Part model, mm, in its own coordinate system. A direction names the side the tool comes from. Round coordinates to 2 decimals unless told otherwise and drop trailing zeros. Loops run counter-clockwise (first coordinate to the right, second up) from the corner with the lowest first, then second, coordinate; pieces in that order, holes last. Notation, with made-up numbers: M -25.5,16.5 L -0.5,16.5 A27 cw -0.5,51.5 Z; hole C 24,45 d11. An arc over 180 degrees is marked long. Put each result on its own line as item: value. Start each with the question number.
1) Slice it at B-B on y = 13.97. State how many separate pieces and enclosed holes the cut face has, then the cut area to 3 significant figures.
2) Probe line 1 along X through (y, z) = (3.5, 145); line 2 along Y through (x, z) = (45, 132.5); line 3 along X through (y, z) = (1.45, 419.1). List the from-to ranges inside material, lowest first.
3) Pull direction Z, two halves, no side cores. Call faces 1 (the flat face through (41.69, 1.25, 8.85)), 2 (the flat face through (25, 2.54, 213)), 3 (the flat face through (26.553, 1.252, 88.849)): +Z half, -Z half, draft (parallel to the pull), parting line (faces both ways), or undercut.
4) Slice it at C-C on z = 76. Give the cut face in (x, y), then the cut area to 3 significant figures.
5) Which spindle directions (+Z, -Z, +X, -X, +Y, -Y) get a long thin tool onto all of the face, cutting with end or side? Do faces 4 (the flat face through (26, 0, 213)), 5 (the flat face through (2.54, 14, 213)), 6 (the flat face through (26.553, 1.252, 355.549)). Say none if no direction does.
6) Slice it at A-A on z = 303. Give the cut face in (x, y), then the cut area to 3 significant figures.
7) Slice it at D-D on z = 169.5. Give the cut face in (x, y), then the cut area to 3 significant figures.
8) Drop flat-ended pins along their axis: pin 1 Ø12 at (x, y) = (45, 9) entering from -Z; pin 2 Ø10 at (x, z) = (44.5, 307) entering from -Y; pin 3 Ø1.3 at (x, y) = (17, 1.5) entering from -Z; pin 4 Ø8 at (x, y) = (9.5, 6) entering from +Z. Give the stop position or say it passes through.
```python
from build123d import *

# Parameters (mm, degrees)
BOSS_EXTRUDE1_DEPTH   = 431.8
SKETCH2_W             = 50.8
SKETCH2_H             = 38.1
TABS_DEPTH            = 22.86
HOLES_REACH           = 4.54
SKETCH3_R             = 2.5796875
SLOTS_DEPTH           = 51.8
TRIG_HOLES_REACH      = 27.4
TAB_CORNER_CUTS_REACH = 27.4


with BuildPart() as part:
    # Sketch1 → Boss-Extrude1 (new body)
    with BuildSketch(Plane.XY):
        Polygon((48.26, 2.54), (48.26, 25.4), (50.8, 25.4), (50.8, 0), (0, 0), (0, 25.4), (2.54, 25.4), (2.54, 2.54), align=None)
    extrude(amount=BOSS_EXTRUDE1_DEPTH)

    # Sketch2 → Tabs (cut)
    with BuildSketch(Plane(origin=(0, 25.4, 0), x_dir=(1, 0, 0), z_dir=(0, 1, 0))):
        with Locations((25.4, -412.75)):
            Rectangle(SKETCH2_W, SKETCH2_H)
        with Locations((25.4, -19.05)):
            Rectangle(SKETCH2_W, SKETCH2_H)
    extrude(amount=-TABS_DEPTH, mode=Mode.SUBTRACT)

    # Sketch3 → Holes (cut, up to next)
    with BuildSketch(Plane(origin=(0, 2.54, 0), x_dir=(1, 0, 0), z_dir=(0, 1, 0)), mode=Mode.PRIVATE) as holes_sk1:
        with Locations((25.4, -419.1)):
            Circle(SKETCH3_R)
    holes_tool1 = extrude(holes_sk1.sketch, amount=-HOLES_REACH, mode=Mode.PRIVATE) & part.part
    add(holes_tool1.solids().sort_by_distance((25.4, 2.54, 419.1))[0], mode=Mode.SUBTRACT)
    # Sketch3 → Holes (cut, up to next)
    with BuildSketch(Plane(origin=(0, 2.54, 0), x_dir=(1, 0, 0), z_dir=(0, 1, 0)), mode=Mode.PRIVATE) as holes_sk2:
        with Locations((25.4, -12.7)):
            Circle(SKETCH3_R)
    holes_tool2 = extrude(holes_sk2.sketch, amount=-HOLES_REACH, mode=Mode.PRIVATE) & part.part
    add(holes_tool2.solids().sort_by_distance((25.4, 2.54, 12.7))[0], mode=Mode.SUBTRACT)

    # Sketch4 → Slots (cut, through all)
    with BuildSketch(Plane(origin=(50.8, 0, 0), x_dir=(0, 0, -1), z_dir=(1, 0, 0))):
        with BuildLine():
            Line((-57.15, 7.62), (-117.475, 7.62))
            ThreePointArc((-117.475, 7.62), (-123.825, 13.97), (-117.475, 20.32))
            Line((-117.475, 20.32), (-57.15, 20.32))
            ThreePointArc((-57.15, 20.32), (-50.8, 13.97), (-57.15, 7.62))
        make_face()
        with BuildLine():
            Line((-142.875, 7.62), (-203.2, 7.62))
            ThreePointArc((-203.2, 7.62), (-209.55, 13.97), (-203.2, 20.32))
            Line((-203.2, 20.32), (-142.875, 20.32))
            ThreePointArc((-142.875, 20.32), (-136.525, 13.97), (-142.875, 7.62))
        make_face()
        with BuildLine():
            Line((-228.6, 7.62), (-288.925, 7.62))
            ThreePointArc((-288.925, 7.62), (-295.275, 13.97), (-288.925, 20.32))
            Line((-288.925, 20.32), (-228.6, 20.32))
            ThreePointArc((-228.6, 20.32), (-222.25, 13.97), (-228.6, 7.62))
        make_face()
        with BuildLine():
            Line((-314.325, 7.62), (-374.65, 7.62))
            ThreePointArc((-374.65, 7.62), (-381, 13.97), (-374.65, 20.32))
            Line((-374.65, 20.32), (-314.325, 20.32))
            ThreePointArc((-314.325, 20.32), (-307.975, 13.97), (-314.325, 7.62))
        make_face()
    extrude(amount=-SLOTS_DEPTH, mode=Mode.SUBTRACT)

    # Sketch5 → Trig_Holes (cut, up to next)
    with BuildSketch(Plane.XZ, mode=Mode.PRIVATE) as trig_holes_sk1:
        with BuildLine():
            Line((41.275, 52.3875), (12.7, 52.3875))
            ThreePointArc((12.7, 52.3875), (9.860193669, 54.142596834), (10.16, 57.4675))
            Line((10.16, 57.4675), (38.735, 95.5675))
            ThreePointArc((38.735, 95.5675), (42.279023157, 96.674569471), (44.45, 93.6625))
            Line((44.45, 93.6625), (44.45, 55.5625))
            ThreePointArc((44.45, 55.5625), (43.52006403, 53.31743597), (41.275, 52.3875))
        make_face()
    trig_holes_tool1 = extrude(trig_holes_sk1.sketch, amount=-TRIG_HOLES_REACH, mode=Mode.PRIVATE) & part.part
    add(trig_holes_tool1.solids().sort_by_distance((31.731608, 0, 68.958649))[0], mode=Mode.SUBTRACT)
    # Sketch5 → Trig_Holes (cut, up to next)
    with BuildSketch(Plane.XZ, mode=Mode.PRIVATE) as trig_holes_sk2:
        with BuildLine():
            Line((9.525, 112.7125), (38.1, 112.7125))
            ThreePointArc((38.1, 112.7125), (40.939806331, 110.957403166), (40.64, 107.6325))
            Line((40.64, 107.6325), (12.065, 69.5325))
            ThreePointArc((12.065, 69.5325), (8.520976843, 68.425430529), (6.35, 71.4375))
            Line((6.35, 71.4375), (6.35, 109.5375))
            ThreePointArc((6.35, 109.5375), (7.27993597, 111.78256403), (9.525, 112.7125))
        make_face()
    trig_holes_tool2 = extrude(trig_holes_sk2.sketch, amount=-TRIG_HOLES_REACH, mode=Mode.PRIVATE) & part.part
    add(trig_holes_tool2.solids().sort_by_distance((19.068392, 0, 96.141351))[0], mode=Mode.SUBTRACT)
    # Sketch5 → Trig_Holes (cut, up to next)
    with BuildSketch(Plane.XZ, mode=Mode.PRIVATE) as trig_holes_sk3:
        with BuildLine():
            Line((41.275, 119.0625), (12.7, 119.0625))
            ThreePointArc((12.7, 119.0625), (9.860193669, 120.817596834), (10.16, 124.1425))
            Line((10.16, 124.1425), (38.735, 162.2425))
            ThreePointArc((38.735, 162.2425), (42.279023157, 163.349569471), (44.45, 160.3375))
            Line((44.45, 160.3375), (44.45, 122.2375))
            ThreePointArc((44.45, 122.2375), (43.52006403, 119.99243597), (41.275, 119.0625))
        make_face()
    trig_holes_tool3 = extrude(trig_holes_sk3.sketch, amount=-TRIG_HOLES_REACH, mode=Mode.PRIVATE) & part.part
    add(trig_holes_tool3.solids().sort_by_distance((31.731608, 0, 135.633649))[0], mode=Mode.SUBTRACT)
    # Sketch5 → Trig_Holes (cut, up to next)
    with BuildSketch(Plane.XZ, mode=Mode.PRIVATE) as trig_holes_sk4:
        with BuildLine():
            Line((9.525, 179.3875), (38.1, 179.3875))
            ThreePointArc((38.1, 179.3875), (40.939806331, 177.632403166), (40.64, 174.3075))
            Line((40.64, 174.3075), (12.065, 136.2075))
            ThreePointArc((12.065, 136.2075), (8.520976843, 135.100430529), (6.35, 138.1125))
            Line((6.35, 138.1125), (6.35, 176.2125))
            ThreePointArc((6.35, 176.2125), (7.27993597, 178.45756403), (9.525, 179.3875))
        make_face()
    trig_holes_tool4 = extrude(trig_holes_sk4.sketch, amount=-TRIG_HOLES_REACH, mode=Mode.PRIVATE) & part.part
    add(trig_holes_tool4.solids().sort_by_distance((19.068392, 0, 162.816351))[0], mode=Mode.SUBTRACT)
    # Sketch5 → Trig_Holes (cut, up to next)
    with BuildSketch(Plane.XZ, mode=Mode.PRIVATE) as trig_holes_sk5:
        with BuildLine():
            Line((41.275, 185.7375), (12.7, 185.7375))
            ThreePointArc((12.7, 185.7375), (9.860193669, 187.492596834), (10.16, 190.8175))
            Line((10.16, 190.8175), (38.735, 228.9175))
            ThreePointArc((38.735, 228.9175), (42.279023157, 230.024569471), (44.45, 227.0125))
            Line((44.45, 227.0125), (44.45, 188.9125))
            ThreePointArc((44.45, 188.9125), (43.52006403, 186.66743597), (41.275, 185.7375))
        make_face()
    trig_holes_tool5 = extrude(trig_holes_sk5.sketch, amount=-TRIG_HOLES_REACH, mode=Mode.PRIVATE) & part.part
    add(trig_holes_tool5.solids().sort_by_distance((31.731608, 0, 202.308649))[0], mode=Mode.SUBTRACT)
    # Sketch5 → Trig_Holes (cut, up to next)
    with BuildSketch(Plane.XZ, mode=Mode.PRIVATE) as trig_holes_sk6:
        with BuildLine():
            Line((9.525, 246.0625), (38.1, 246.0625))
            ThreePointArc((38.1, 246.0625), (40.939806331, 244.307403166), (40.64, 240.9825))
            Line((40.64, 240.9825), (12.065, 202.8825))
            ThreePointArc((12.065, 202.8825), (8.520976843, 201.775430529), (6.35, 204.7875))
            Line((6.35, 204.7875), (6.35, 242.8875))
            ThreePointArc((6.35, 242.8875), (7.27993597, 245.13256403), (9.525, 246.0625))
        make_face()
    trig_holes_tool6 = extrude(trig_holes_sk6.sketch, amount=-TRIG_HOLES_REACH, mode=Mode.PRIVATE) & part.part
    add(trig_holes_tool6.solids().sort_by_distance((19.068392, 0, 229.491351))[0], mode=Mode.SUBTRACT)
    # Sketch5 → Trig_Holes (cut, up to next)
    with BuildSketch(Plane.XZ, mode=Mode.PRIVATE) as trig_holes_sk7:
        with BuildLine():
            Line((41.275, 252.4125), (12.7, 252.4125))
            ThreePointArc((12.7, 252.4125), (9.860193669, 254.167596834), (10.16, 257.4925))
            Line((10.16, 257.4925), (38.735, 295.5925))
            ThreePointArc((38.735, 295.5925), (42.279023157, 296.699569471), (44.45, 293.6875))
            Line((44.45, 293.6875), (44.45, 255.5875))
            ThreePointArc((44.45, 255.5875), (43.52006403, 253.34243597), (41.275, 252.4125))
        make_face()
    trig_holes_tool7 = extrude(trig_holes_sk7.sketch, amount=-TRIG_HOLES_REACH, mode=Mode.PRIVATE) & part.part
    add(trig_holes_tool7.solids().sort_by_distance((31.731608, 0, 268.983649))[0], mode=Mode.SUBTRACT)
    # Sketch5 → Trig_Holes (cut, up to next)
    with BuildSketch(Plane.XZ, mode=Mode.PRIVATE) as trig_holes_sk8:
        with BuildLine():
            Line((9.525, 312.7375), (38.1, 312.7375))
            ThreePointArc((38.1, 312.7375), (40.939806331, 310.982403166), (40.64, 307.6575))
            Line((40.64, 307.6575), (12.065, 269.5575))
            ThreePointArc((12.065, 269.5575), (8.520976843, 268.450430529), (6.35, 271.4625))
            Line((6.35, 271.4625), (6.35, 309.5625))
            ThreePointArc((6.35, 309.5625), (7.27993597, 311.80756403), (9.525, 312.7375))
        make_face()
    trig_holes_tool8 = extrude(trig_holes_sk8.sketch, amount=-TRIG_HOLES_REACH, mode=Mode.PRIVATE) & part.part
    add(trig_holes_tool8.solids().sort_by_distance((19.068392, 0, 296.166351))[0], mode=Mode.SUBTRACT)
    # Sketch5 → Trig_Holes (cut, up to next)
    with BuildSketch(Plane.XZ, mode=Mode.PRIVATE) as trig_holes_sk9:
        with BuildLine():
            Line((41.275, 319.0875), (12.7, 319.0875))
            ThreePointArc((12.7, 319.0875), (9.860193669, 320.842596834), (10.16, 324.1675))
            Line((10.16, 324.1675), (38.735, 362.2675))
            ThreePointArc((38.735, 362.2675), (42.279023157, 363.374569471), (44.45, 360.3625))
            Line((44.45, 360.3625), (44.45, 322.2625))
            ThreePointArc((44.45, 322.2625), (43.52006403, 320.01743597), (41.275, 319.0875))
        make_face()
    trig_holes_tool9 = extrude(trig_holes_sk9.sketch, amount=-TRIG_HOLES_REACH, mode=Mode.PRIVATE) & part.part
    add(trig_holes_tool9.solids().sort_by_distance((31.731608, 0, 335.658649))[0], mode=Mode.SUBTRACT)
    # Sketch5 → Trig_Holes (cut, up to next)
    with BuildSketch(Plane.XZ, mode=Mode.PRIVATE) as trig_holes_sk10:
        with BuildLine():
            Line((9.525, 379.4125), (38.1, 379.4125))
            ThreePointArc((38.1, 379.4125), (40.939806331, 377.657403166), (40.64, 374.3325))
            Line((40.64, 374.3325), (12.065, 336.2325))
            ThreePointArc((12.065, 336.2325), (8.520976843, 335.125430529), (6.35, 338.1375))
            Line((6.35, 338.1375), (6.35, 376.2375))
            ThreePointArc((6.35, 376.2375), (7.27993597, 378.48256403), (9.525, 379.4125))
        make_face()
    trig_holes_tool10 = extrude(trig_holes_sk10.sketch, amount=-TRIG_HOLES_REACH, mode=Mode.PRIVATE) & part.part
    add(trig_holes_tool10.solids().sort_by_distance((19.068392, 0, 362.841351))[0], mode=Mode.SUBTRACT)

    # Sketch6 → Tab_Corner_Cuts (cut, up to next)
    with BuildSketch(Plane.XZ, mode=Mode.PRIVATE) as tab_corner_cuts_sk1:
        Polygon((32.839487758, 0), (50.8, 17.960512242), (50.8, 0), align=None)
    tab_corner_cuts_tool1 = extrude(tab_corner_cuts_sk1.sketch, amount=-TAB_CORNER_CUTS_REACH, mode=Mode.PRIVATE) & part.part
    add(tab_corner_cuts_tool1.solids().sort_by_distance((44.813163, 0, 5.986837))[0], mode=Mode.SUBTRACT)
    # Sketch6 → Tab_Corner_Cuts (cut, up to next)
    with BuildSketch(Plane.XZ, mode=Mode.PRIVATE) as tab_corner_cuts_sk2:
        Polygon((17.960512242, 0), (0, 17.960512242), (0, 0), align=None)
    tab_corner_cuts_tool2 = extrude(tab_corner_cuts_sk2.sketch, amount=-TAB_CORNER_CUTS_REACH, mode=Mode.PRIVATE) & part.part
    add(tab_corner_cuts_tool2.solids().sort_by_distance((5.986837, 0, 5.986837))[0], mode=Mode.SUBTRACT)
    # Sketch6 → Tab_Corner_Cuts (cut, up to next)
    with BuildSketch(Plane.XZ, mode=Mode.PRIVATE) as tab_corner_cuts_sk3:
        Polygon((32.839487758, 431.8), (50.8, 413.839487758), (50.8, 431.8), align=None)
    tab_corner_cuts_tool3 = extrude(tab_corner_cuts_sk3.sketch, amount=-TAB_CORNER_CUTS_REACH, mode=Mode.PRIVATE) & part.part
    add(tab_corner_cuts_tool3.solids().sort_by_distance((44.813163, 0, 425.813163))[0], mode=Mode.SUBTRACT)
    # Sketch6 → Tab_Corner_Cuts (cut, up to next)
    with BuildSketch(Plane.XZ, mode=Mode.PRIVATE) as tab_corner_cuts_sk4:
        Polygon((17.960512242, 431.8), (0, 413.839487758), (0, 431.8), align=None)
    tab_corner_cuts_tool4 = extrude(tab_corner_cuts_sk4.sketch, amount=-TAB_CORNER_CUTS_REACH, mode=Mode.PRIVATE) & part.part
    add(tab_corner_cuts_tool4.solids().sort_by_distance((5.986837, 0, 425.813163))[0], mode=Mode.SUBTRACT)


solid = part.part
```
Recorded:
1. separate pieces: 10
1. enclosed holes: 0
1. area: 323 mm2
2. line 1: x = 0 to 2.54, 48.26 to 50.8
2. line 2: y = 0 to 2.54
2. line 3: x = 5.26 to 22.82, 27.98 to 45.54
3. face 1: -Z half
3. face 2: draft
3. face 3: undercut
4. outline: M 0,0 L 6.35,0 L 6.35,2.54 L 2.54,2.54 L 2.54,7.62 L 0,7.62 Z; M 0,20.32 L 2.54,20.32 L 2.54,25.4 L 0,25.4 Z; M 16.92,0 L 24.06,0 L 24.06,2.54 L 16.92,2.54 Z; M 44.45,0 L 50.8,0 L 50.8,7.62 L 48.26,7.62 L 48.26,2.54 L 44.45,2.54 Z; M 48.26,20.32 L 50.8,20.32 L 50.8,25.4 L 48.26,25.4 Z
4. area: 102 mm2
5. face 4: +Z, -Z, +X, -X, -Y
5. face 5: +Z, -Z, +Y
5. face 6: +Y, -Y
6. outline: M 0,0 L 6.35,0 L 6.35,2.54 L 2.54,2.54 L 2.54,25.4 L 0,25.4 Z; M 37.15,0 L 50.8,0 L 50.8,25.4 L 48.26,25.4 L 48.26,2.54 L 37.15,2.54 Z
6. area: 167 mm2
7. outline: M 0,0 L 6.35,0 L 6.35,2.54 L 2.54,2.54 L 2.54,7.62 L 0,7.62 Z; M 0,20.32 L 2.54,20.32 L 2.54,25.4 L 0,25.4 Z; M 37.03,0 L 50.8,0 L 50.8,7.62 L 48.26,7.62 L 48.26,2.54 L 37.03,2.54 Z; M 48.26,20.32 L 50.8,20.32 L 50.8,25.4 L 48.26,25.4 Z
7. area: 103 mm2
8. pin 1: stops at z = 38.1
8. pin 2: stops at y = 0
8. pin 3: stops at z = 0.31
8. pin 4: stops at z = 425.35
